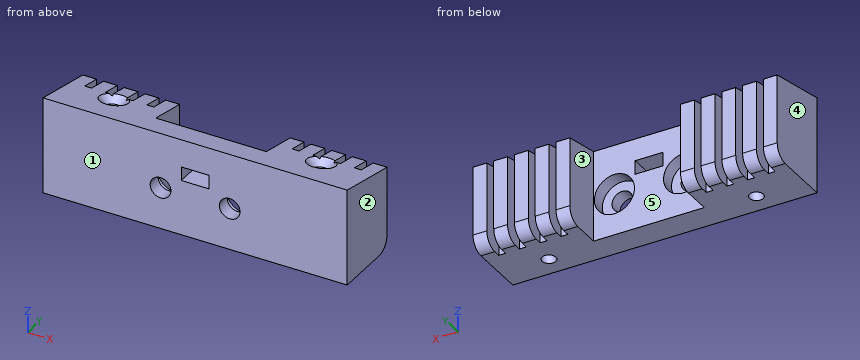
from build123d import *

# Parameters (mm, degrees)
F1_DEPTH        = 22
F2_W            = 16
F2_H            = 12
F2_H_2          = 2
F3_DEPTH        = 6
F4_W            = 1
F4_H            = 14
F4_H_2          = 12
F4_H_3          = 2
F5_DEPTH        = 3
F6_R            = 2
F8_D            = 2
F8_DEPTH        = 15
F8_CSINK_D      = 4
F8_CSINK_ANGLE  = 90
F8_TIP          = 0.600860619
F9_W            = 4
F9_H            = 2
F10_DEPTH       = 25
F11_D           = 3
F11_DEPTH       = 15
F11_CBORE_D     = 5.8
F11_CBORE_DEPTH = 2
F11_TIP         = 0.9012909285


with BuildPart() as f1:
    # F0 (on Right) → F1 (new body, symmetric)
    with BuildSketch(Plane.YZ):
        Polygon((-5, -7), (5, -7), (5, 5), (-5, 7), align=None)
    extrude(amount=F1_DEPTH, both=True)

    # F2 (on face) → F3 (cut)
    with BuildSketch(Plane(origin=(0, 5, 0), x_dir=(-1, 0, 0), z_dir=(0, 1, 0))):
        with Locations((0, -1)):
            Rectangle(F2_W, F2_H)
        with Locations((0, 6)):
            Rectangle(F2_W, F2_H_2)
    extrude(amount=-F3_DEPTH, mode=Mode.SUBTRACT)

    # F4 (on face) → F5 (cut)
    with BuildSketch(Plane(origin=(0, 5, 0), x_dir=(-1, 0, 0), z_dir=(0, 1, 0))):
        with Locations((-10.5, 0)):
            Rectangle(F4_W, F4_H)
        with Locations((-13.5, 0)):
            Rectangle(F4_W, F4_H)
        with Locations((-16.5, 0)):
            Rectangle(F4_W, F4_H)
        with Locations((-19.5, 0)):
            Rectangle(F4_W, F4_H)
        with Locations((10.5, -1)):
            Rectangle(F4_W, F4_H_2)
        with Locations((13.5, -1)):
            Rectangle(F4_W, F4_H_2)
        with Locations((16.5, -1)):
            Rectangle(F4_W, F4_H_2)
        with Locations((19.5, -1)):
            Rectangle(F4_W, F4_H_2)
        with Locations((19.5, 6)):
            Rectangle(F4_W, F4_H_3)
        with Locations((16.5, 6)):
            Rectangle(F4_W, F4_H_3)
        with Locations((13.5, 6)):
            Rectangle(F4_W, F4_H_3)
        with Locations((10.5, 6)):
            Rectangle(F4_W, F4_H_3)
    extrude(amount=-F5_DEPTH, mode=Mode.SUBTRACT)

    # F6
    f6_edges = [f1.edges().sort_by_distance(p)[0] for p in [
        (21, 5, -7),
        (18, 5, -7),
        (15, 5, -7),
        (12, 5, -7),
        (9, 5, -7),
        (-9, 5, -7),
        (-12, 5, -7),
        (-15, 5, -7),
        (-18, 5, -7),
        (-21, 5, -7),
    ]]
    fillet(f6_edges, radius=F6_R)

    # F8
    with Locations(Plane(origin=(0, 1.1538461538, 5.7692307692), x_dir=(1, 0, 0), z_dir=(0, 0.1961161351, 0.9805806757))):
        with Locations((15, -0.5257163244), (-15, -0.5257163244)):
            CounterSinkHole(F8_D / 2, F8_CSINK_D / 2, depth=F8_DEPTH, counter_sink_angle=F8_CSINK_ANGLE)
            with Locations((0, 0, -(F8_DEPTH + F8_TIP / 2))):  # 118° drill point
                Cone(0, F8_D / 2, F8_TIP, mode=Mode.SUBTRACT)

    # F9 (on face) → F10 (cut)
    with BuildSketch(Plane(origin=(0, -1, 0), x_dir=(-1, 0, 0), z_dir=(0, 1, 0))):
        with Locations((0, 2)):
            Rectangle(F9_W, F9_H)
    extrude(amount=-F10_DEPTH, mode=Mode.SUBTRACT)

    # F11
    with Locations(Plane(origin=(0, -1, 0), x_dir=(-1, 0, 0), z_dir=(0, 1, 0))):
        with Locations((-5, -1), (5, -1)):
            CounterBoreHole(F11_D / 2, F11_CBORE_D / 2, F11_CBORE_DEPTH, depth=F11_DEPTH)
            with Locations((0, 0, -(F11_DEPTH + F11_TIP / 2))):  # 118° drill point
                Cone(0, F11_D / 2, F11_TIP, mode=Mode.SUBTRACT)


solid = f1.part
Could you check a few things on this model? Use its own coordinates, in mm. Face numbers are marked on the shaded views. A direction names the side the tool comes from. Round coordinates to 2 decimals unless told otherwise and drop trailing zeros. Order: outer loops, then holes, each group sorted by start corner. A loop starts at its lowest first (then second) coordinate and runs counter-clockwise, first axis right, second up.
(1) Imagine slicing it at C-C (x = -4). Write out the boundary of the cut face in (y, z).
Response values:
outline: (-5, -7) - (-1, -7) - (-1, -3.72) - (-3, -3.72) - (-3, -2.12) - (-5, -2.12) - close; (-5, 0.12) - (-3, 0.12) - (-3, 1.72) - (-1, 1.72) - (-1, 6.2) - (-5, 7) - close
(2) Imagine slicing it at A-A (y = -3.75). Write out the boundary of the cut face in (x, z).
Response values:
outline: (-22, -7) - (22, -7) - (22, 6.75) - (-22, 6.75) - close; hole circle Ø3 at (-5, -1); hole (-2, 1) - (2, 1) - (2, 3) - (-2, 3) - close; hole circle Ø3 at (5, -1)
(3) I'm going to push flat-ended pins straight in: pin 1 (0.8 mm diameter, centred on x = 19.5, z = 1, fed in from +Y); pin 2 (1 mm diameter, centred on x = 0.5, z = 0.5, fed in from +Y); pin 3 (5 mm diameter, centred on x = -5, z = -1, fed in from +Y). Where does each tip first touch, or does it pass through?
Response values:
pin 1: stops at y = 2
pin 2: stops at y = -1
pin 3: stops at y = -3
(4) Imagine slicing it at D-D (z = 1.5). Count the separate pieces of the cut face and the enclosed holes in it, plus the area to 3 significant figures.
Response values:
separate pieces: 2
enclosed holes: 2
area: 286 mm2
(5) If we mould it in two halves opening along X, with no side actions, what happens to the marked faces 1, 2 and 3? For each: released by +X, released by -X, zero draft, split by the parting line, or undercut.
Response values:
face 1: zero draft
face 2: released by +X
face 3: undercut
(6) Please list where these lines run through material, in increasing order: line 1 along X through (y, z) = (-0.75, -1.25); line 2 along X through (y, z) = (-3.5, 0); line 3 along Z through (x, y) = (5, -4.1).
Response values:
line 1: x = -22 to -16, -14 to -8, 8 to 14, 16 to 22
line 2: x = -22 to -6.12, -3.88 to 3.88, 6.12 to 22
line 3: z = -7 to -2.5, 0.5 to 6.82
(7) Imagine slicing it at B-B (x = 5). Write out the boundary of the cut face in (y, z), plus the area to 3 significant figures.
Response values:
outline: (-5, -7) - (-1, -7) - (-1, -3.9) - (-3, -3.9) - (-3, -2.5) - (-5, -2.5) - close; (-5, 0.5) - (-3, 0.5) - (-3, 1.9) - (-1, 1.9) - (-1, 6.2) - (-5, 7) - close
area: 36.8 mm2
(8) Which directions (+Z, -Z, +X, -X, +Y, -Y) give clear straight access to the entire face, cutting with the end or side of a thin tool? Please do the marked faces 4 and 5.
Response values:
face 4: +Z, -Z, -X, +Y, -Y
face 5: +Z, -Z, +Y
